from build123d import *

# Parameters (mm, degrees)
BOSS_EXTRUDE1_DEPTH             = 11.5
F_2_56_TAPPED_HOLE3_D           = 1.778
F_2_56_TAPPED_HOLE3_CSINK_D     = 3.4544
F_2_56_TAPPED_HOLE3_CSINK_ANGLE = 90
CUT_EXTRUDE1_DEPTH              = 10
F_2_56_TAPPED_HOLE1_D           = 1.778
F_2_56_TAPPED_HOLE1_CSINK_D     = 3.4544
F_2_56_TAPPED_HOLE1_CSINK_ANGLE = 90
BOSS_EXTRUDE2_DEPTH             = 10
F_2_56_TAPPED_HOLE4_D           = 1.778
F_2_56_TAPPED_HOLE4_CSINK_D     = 3.4544
F_2_56_TAPPED_HOLE4_CSINK_ANGLE = 90
F_2_CLEARANCE_HOLE1_D           = 2.4384


with BuildPart() as part:
    # Sketch1 → Boss-Extrude1 (new body, symmetric)
    with BuildSketch(Plane.XY):
        with BuildLine():
            Line((-10, 39.778288752), (-10, 51.016))
            Line((-10, 51.016), (10, 51.016))
            Line((10, 51.016), (10, 39.778288752))
            ThreePointArc((10, 39.778288752), (0, 41.016), (-10, 39.778288752))
        make_face()
    extrude(amount=BOSS_EXTRUDE1_DEPTH, both=True)

    # #2-56 Tapped Hole3 (through all)
    with Locations(Plane(origin=(0, 51.016, 0), x_dir=(1, 0, 0), z_dir=(0, 1, 0))):
        with Locations((0, -1.5)):
            CounterSinkHole(F_2_56_TAPPED_HOLE3_D / 2, F_2_56_TAPPED_HOLE3_CSINK_D / 2, counter_sink_angle=F_2_56_TAPPED_HOLE3_CSINK_ANGLE)

    # Sketch2 → Cut-Extrude1 (cut, symmetric)
    with BuildSketch(Plane(origin=(0, 0, 0), x_dir=(0, 0, -1), z_dir=(1, 0, 0))):
        Polygon((-11.5, 45.307541641), (11.5, 49.778288752), (11.5, 51.016), (-11.5, 51.016), align=None)
    extrude(amount=CUT_EXTRUDE1_DEPTH, both=True, mode=Mode.SUBTRACT)

    # #2-56 Tapped Hole1 (through all)
    with Locations(Plane(origin=(0, 45.811969283, 8.904944751), x_dir=(1, 0, 0), z_dir=(0, 0.981627183, 0.190808995))):
        with Locations((6.5, 1.356373894), (6.5, 13.356373894), (-6.5, 13.356373894), (-6.5, 1.356373894)):
            CounterSinkHole(F_2_56_TAPPED_HOLE1_D / 2, F_2_56_TAPPED_HOLE1_CSINK_D / 2, counter_sink_angle=F_2_56_TAPPED_HOLE1_CSINK_ANGLE)

    # Sketch5 → Boss-Extrude2 (add)
    with BuildSketch(Plane(origin=(0, 0, -11.5), x_dir=(-1, 0, 0), z_dir=(0, 0, -1))):
        with BuildLine():
            Line((10, 39.778288752), (10, 49.778288752))
            Line((10, 49.778288752), (-10, 49.778288752))
            Line((-10, 49.778288752), (-10, 39.778288752))
            ThreePointArc((-10, 39.778288752), (0, 41.016), (10, 39.778288752))
        make_face()
    extrude(amount=BOSS_EXTRUDE2_DEPTH)

    # #2-56 Tapped Hole4 (through all)
    with Locations(Plane(origin=(0, 49.778288752, 0), x_dir=(1, 0, 0), z_dir=(0, 1, 0))):
        with Locations((0, 13.5)):
            CounterSinkHole(F_2_56_TAPPED_HOLE4_D / 2, F_2_56_TAPPED_HOLE4_CSINK_D / 2, counter_sink_angle=F_2_56_TAPPED_HOLE4_CSINK_ANGLE)

    # #2 Clearance Hole1 (through all)
    with Locations(Plane.ZY.offset(10)):
        with Locations((-17.5, 44.778288752)):
            Hole(F_2_CLEARANCE_HOLE1_D / 2)


solid = part.part
The listing builds one solid part. Answer for the finished solid, in the listing's coordinates (mm). Give positions to 0.01 mm unless a question says otherwise; leave off trailing zeros. Loops run counter-clockwise (first coordinate to the right, second up) from the corner with the lowest first, then second, coordinate; pieces in that order, holes last. Notation, with made-up numbers: (48, 81) - (66, 81) arc R16 ccw to (66, 86) - close; hole circle Ø11 at (71, 62.25). An arc over 180 degrees is marked (long way). Answer as a JSON object with one key per item and string values.
1. A cutting plane is placed at B-B (x = 0). Write down the section's boundary in (y, z).
Determined:
{"outline": "(41.02, -21.5) - (49.78, -21.5) - (49.78, -15.23) - (48.94, -14.39) - (41.02, -14.39) - close; (41.02, -12.61) - (48.94, -12.61) - (49.78, -11.77) - (49.78, -11.5) - (47.42, 0.61) - (41.02, 0.61) - close; (41.02, 2.39) - (47.08, 2.39) - (45.31, 11.5) - (41.02, 11.5) - close; hole circle Ø2.44 at (44.78, -17.5)"}
2. For a pull along X with two mould halves and no side action, classify faces 1 (the flat face through (-10, 44, -5)), 2 (the flat face through (10, 44, -5)), 3 (the cylindrical face through (0.141, 41.016, -4.769)) as pulls with the +X half, pulls with the -X half, needs draft (parallel to the pull), parting line crosses it, or undercut.
Determined:
{"face 1": "pulls with the -X half", "face 2": "pulls with the +X half", "face 3": "undercut"}
3. Flat-ended cylindrical pins translate along their axes: pin 1 Ø2 at (y, z) = (44.78, -17.5) entering from +X; pin 2 Ø3 at (x, y) = (-3, 46.5) entering from +Z; pin 3 Ø2 at (x, z) = (0, 1.5) entering from +Y; pin 4 Ø2 at (x, z) = (0, -13.5) entering from -Y. Find the tip coordinate at first contact, or state that the pin passes through.
Determined:
{"pin 1": "through", "pin 2": "z = 11.5", "pin 3": "y = 47.45", "pin 4": "y = 41"}
4. Find the intervals of material crossed by L1, parallel to X at y = 45.25, z = -13.5; L2, parallel to Z at x = 0.75, y = 44; L3, parallel to Y at x = 1, z = -17.5, in increasing order. Write a range as [from, to].
Determined:
{"L1": "[-10, -0.89], [0.89, 10]", "L2": "[-21.5, -18.44], [-16.56, -13.98], [-13.02, 1.02], [1.98, 11.5]", "L3": "[41, 43.56], [46, 49.78]"}
5. A cutting plane is placed at C-C (z = -13.5). Write down the section's boundary in (x, y), then the cut area to 3 significant figures.
Determined:
{"outline": "(-10, 39.78) arc R41.02 cw to (-0.89, 41.01) - (-0.89, 48.94) - (-1.73, 49.78) - (-10, 49.78) - close; (0.89, 41.01) arc R41.02 cw to (10, 39.78) - (10, 49.78) - (1.73, 49.78) - (0.89, 48.94) - close", "area": "167 mm²"}
6. A cutting plane is placed at D-D (y = 44.25). Give the number of separate pieces and of enclosed holes in the cut face, then the cut area to 3 significant figures.
Determined:
{"separate pieces": "2", "enclosed holes": "6", "area": "601 mm²"}
7. A cutting plane is placed at A-A (z = -17.5). Write down the section's boundary in (x, y).
Determined:
{"outline": "(-10, 39.78) arc R41.02 cw to (10, 39.78) - (10, 43.56) - (-10, 43.56) - close; (-10, 46) - (10, 46) - (10, 49.78) - (-10, 49.78) - close"}
